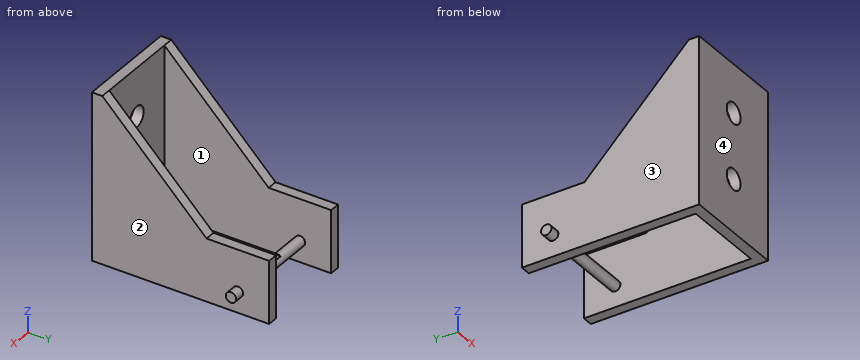
from build123d import *

# Parameters (mm, degrees)
SKETCH2_W                = 63.5
SKETCH2_H                = 6.35
BASE_DEPTH               = 101.6
RIB_DEPTH                = 6.35
CUT_EXTRUDE1_DEPTH       = 159.876949241
CUT_EXTRUDE1_DEPTH_BACK  = 159.876949241
SKETCH5_R                = 3.175
BOSS_EXTRUDE1_DEPTH      = 63.5
BOSS_EXTRUDE1_DEPTH_BACK = 12.7
SKETCH5_2_R              = 3.175
CUT_EXTRUDE2_REACH       = 161.763
SKETCH6_R                = 6.35
SKETCH7_W                = 9.883303814
SKETCH7_H                = 2.121203366
CUT_EXTRUDE3_DEPTH       = 25.4


with BuildPart() as part:
    # Sketch2 → Base (new body)
    with BuildSketch(Plane.XY):
        with Locations((31.75, 3.175)):
            Rectangle(SKETCH2_W, SKETCH2_H)
    extrude(amount=BASE_DEPTH)

    # Sketch4 → Rib (add)
    with BuildSketch(Plane(origin=(63.5, 0, 0), x_dir=(0, 0, -1), z_dir=(1, 0, 0))):
        Polygon((0, 107.95), (0, 6.35), (-101.6, 6.35), (-38.1, 69.85), (-38.1, 107.95), align=None)
    rib = extrude(amount=-RIB_DEPTH)

    # RibCopy: Rib across plane
    add(rib.mirror(Plane.ZY.offset(-31.75)))

    # Sketch5 → Cut-Extrude1 (cut, two sides: drawn at the far end of the back side and taken through both)
    with BuildSketch(Plane.ZY.offset(-57.15).offset(-CUT_EXTRUDE1_DEPTH_BACK)):
        with Locations((12.7, 88.9)):
            Circle(SKETCH5_R)
    extrude(amount=CUT_EXTRUDE1_DEPTH + CUT_EXTRUDE1_DEPTH_BACK, mode=Mode.SUBTRACT)

    # Sketch5_2 → Boss-Extrude1 (add, two sides: drawn at the far end of the back side and taken through both)
    with BuildSketch(Plane.ZY.offset(-57.15).offset(-BOSS_EXTRUDE1_DEPTH_BACK)):
        with Locations((12.7, 88.9)):
            Circle(SKETCH5_2_R)
    extrude(amount=BOSS_EXTRUDE1_DEPTH + BOSS_EXTRUDE1_DEPTH_BACK)

    # Sketch6 → Cut-Extrude2 (cut, up to next)
    with BuildSketch(Plane(origin=(0, 6.35, 0), x_dir=(-1, 0, 0), z_dir=(0, 1, 0)), mode=Mode.PRIVATE) as cut_extrude2_sk1:
        with Locations(Location((-31.75, 72.023550981, 0), (0, 0, 90))):
            Circle(SKETCH6_R)
    cut_extrude2_tool1 = extrude(cut_extrude2_sk1.sketch, amount=-CUT_EXTRUDE2_REACH, mode=Mode.PRIVATE) & part.part
    # Sketch6 → Cut-Extrude2 (cut, up to next)
    with BuildSketch(Plane(origin=(0, 6.35, 0), x_dir=(-1, 0, 0), z_dir=(0, 1, 0)), mode=Mode.PRIVATE) as cut_extrude2_sk2:
        with Locations(Location((-31.75, 32.114477008, 0), (0, 0, 90))):
            Circle(SKETCH6_R)
    cut_extrude2_tool2 = extrude(cut_extrude2_sk2.sketch, amount=-CUT_EXTRUDE2_REACH, mode=Mode.PRIVATE) & part.part
    add(cut_extrude2_tool1.solids().sort_by_distance((31.75, 6.35, 72.023551))[0], mode=Mode.SUBTRACT)
    add(cut_extrude2_tool2.solids().sort_by_distance((31.75, 6.35, 32.114477))[0], mode=Mode.SUBTRACT)

    # Sketch7 → Cut-Extrude3 (cut)
    with BuildSketch(Plane(origin=(0, 107.95, 0), x_dir=(-1, 0, 0), z_dir=(0, 1, 0))):
        with Locations((-32.019903214, 16.271172427)):
            Rectangle(SKETCH7_W, SKETCH7_H)
    extrude(amount=-CUT_EXTRUDE3_DEPTH, mode=Mode.SUBTRACT)


solid = part.part
CAD build for the part. Positions are in the model's coordinates, mm. Face numbers are marked on the shaded views. Coordinates: 2 decimals unless noted, no trailing zeros. Write each loop counter-clockwise with the first axis right and the second up, starting at its lowest first coordinate (ties: lowest second). Pieces come first, ordered by that corner, then holes. Notation, with made-up numbers: (62.5, 60) - (118.5, 60) arc R20 ccw to (118.5, 82) - close; hole circle Ø10 at (38, -32). An arc over 180 degrees is marked (long way). Use a Markdown table: item, result. Add a question column.
Item 1: Band-saw the part on B-B, the plane x = 31.75. Give the cut face in (y, z) (3 decimals).
Item 2: Band-saw the part on D-D, the plane z = 12.7. Give the cut face in (x, y) (3 decimals), and give its area (3 significant figures).
Item 3: Band-saw the part on A-A, the plane y = 75.5. Give the cut face in (x, z), and give its area (3 significant figures).
Item 4: Flat gauge pins, fed straight in: pin 1 (2 mm diameter, centred on y = 34, z = 45.5, fed in from +X); pin 2 (3 mm diameter, centred on x = 32.5, y = 90, fed in from +Z); pin 3 (15 mm diameter, centred on x = 26.5, z = 31, fed in from +Y). Where does each tip first touch, or does it go through?
Item 5: Mould opens along X. For the marked faces 1, 2, 3 and 4 say: pulls with the +X half, pulls with the -X half, needs draft (parallel to the pull), parting line crosses it, or undercut.
Item 6: Drill centre lines: L1, parallel to X at y = 20.5, z = 11.5; L2, parallel to Z at x = 31, y = 2. Where is each one in solid material? Low to high. Write a range as from..to.
Item 7: Band-saw the part on C-C, the plane z = 34.5. Give the cut face in (x, y), and give its area (3 significant figures).
Numbers:
| question | item | result |
|---|---|---|
| 1 | outline | (0, 0) - (6.35, 0) - (6.35, 25.764) - (0, 25.764) - close; (0, 38.464) - (6.35, 38.464) - (6.35, 65.674) - (0, 65.674) - close; (0, 78.374) - (6.35, 78.374) - (6.35, 101.6) - (0, 101.6) - close; (86.956, 15.211) arc R3.175 ccw (long way) to (90.844, 15.211) - close |
| 2 | outline | (-6.35, 85.725) - (0, 85.725) - (0, 0) - (63.5, 0) - (63.5, 85.725) - (69.85, 85.725) - (69.85, 92.075) - (63.5, 92.075) - (63.5, 107.95) - (57.15, 107.95) - (57.15, 92.075) - (6.35, 92.075) - (6.35, 107.95) - (0, 107.95) - (0, 92.075) - (-6.35, 92.075) - close; hole (6.35, 6.35) - (57.15, 6.35) - (57.15, 85.725) - (6.35, 85.725) - close |
| 2 | area | 2,100 mm2 |
| 3 | outline | (0, 0) - (6.35, 0) - (6.35, 38.1) - (0, 38.1) - close; (57.15, 0) - (63.5, 0) - (63.5, 38.1) - (57.15, 38.1) - close |
| 3 | area | 484 mm2 |
| 4 | pin 1 | x = 63.5 |
| 4 | pin 2 | z = 15.21 |
| 4 | pin 3 | y = 6.35 |
| 5 | face 1 | undercut |
| 5 | face 2 | pulls with the +X half |
| 5 | face 3 | pulls with the -X half |
| 5 | face 4 | needs draft |
| 6 | L1 | 0..6.35, 57.15..63.5 |
| 6 | L2 | 0..25.81, 38.42..65.72, 78.33..101.6 |
| 7 | outline | (0, 0) - (25.87, 0) - (25.87, 6.35) - (6.35, 6.35) - (6.35, 107.95) - (0, 107.95) - close; (37.63, 0) - (63.5, 0) - (63.5, 107.95) - (57.15, 107.95) - (57.15, 6.35) - (37.63, 6.35) - close |
| 7 | area | 1,620 mm2 |
